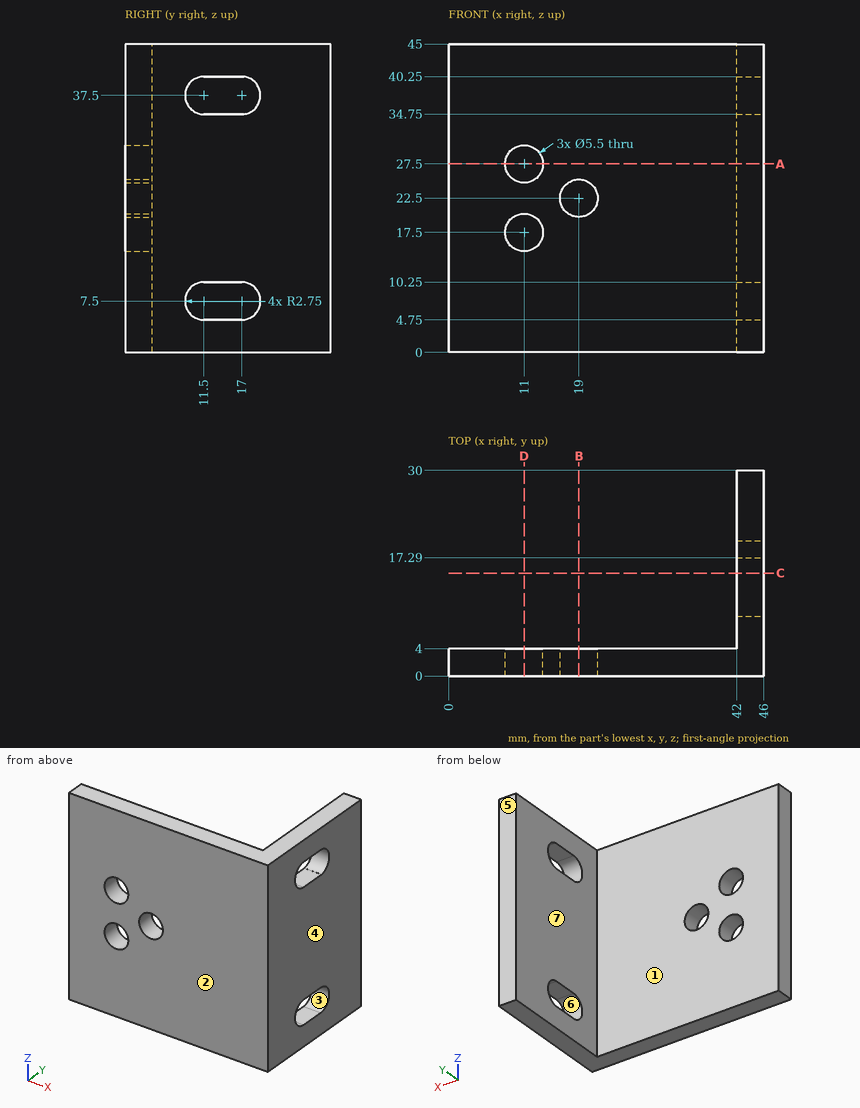
Part print with two shaded views. Sizes in mm from the minimum x, y, z corner. A direction names the side the tool comes from. Coordinates: 2 decimals unless noted, no trailing zeros. Write each loop counter-clockwise with the first axis right and the second up, starting at its lowest first coordinate (ties: lowest second). Pieces come first, ordered by that corner, then holes. Notation, with made-up numbers: M 12,20 L 48,20 A15 cw 48,42 Z; hole C -22.75,-14.5 d9. An arc over 180 degrees is marked long. Return JSON: item names as keys, results as strings.
Item 1: Slice it at B-B, the plane x = 19. Write the cut outline in (y, z), and give its area (3 significant figures).
Findings below:
{"outline": "M 0,0 L 4,0 L 4,19.75 L 0,19.75 Z; M 0,25.25 L 4,25.25 L 4,45 L 0,45 Z", "area": "158 mm2"}
Item 2: Two-plate mould, pull along Y, no slides. Class the marked faces 1, 2, 3 and 4: +Y half, -Y half, draft (parallel to the pull), parting line (faces both ways), or undercut.
Findings below:
{"face 1": "+Y half", "face 2": "-Y half", "face 3": "undercut", "face 4": "draft"}
Item 3: Slice it at C-C, the plane y = 15. Write the cut outline in (x, z).
Findings below:
{"outline": "M 42,0 L 46,0 L 46,4.75 L 42,4.75 Z; M 42,10.25 L 46,10.25 L 46,34.75 L 42,34.75 Z; M 42,40.25 L 46,40.25 L 46,45 L 42,45 Z"}
Item 4: Drop flat-ended pins along their axis: pin 1 Ø1.5 at (y, z) = (20, 27) entering from -X; pin 2 Ø3 at (x, z) = (14, 15.5) entering from +Y. Give the stop position or say it passes through.
Findings below:
{"pin 1": "stops at x = 42", "pin 2": "stops at y = 4"}
Item 5: Which spindle directions (+Z, -Z, +X, -X, +Y, -Y) get a long thin tool onto all of the face, cutting with end or side? Do the marked faces 5, 6 and 7. Say none if no direction does.
Findings below:
{"face 5": "+Z, -Z, +X, -X, +Y", "face 6": "+X, -X", "face 7": "+Z, -Z, -X, +Y"}
Item 6: Slice it at D-D, the plane x = 11. Write the cut outline in (y, z), and give its area (3 significant figures).
Findings below:
{"outline": "M 0,0 L 4,0 L 4,14.75 L 0,14.75 Z; M 0,20.25 L 4,20.25 L 4,24.75 L 0,24.75 Z; M 0,30.25 L 4,30.25 L 4,45 L 0,45 Z", "area": "136 mm2"}
Item 7: Slice it at A-A, the plane z = 27.5. Write the cut outline in (x, y).
Findings below:
{"outline": "M 0,0 L 8.25,0 L 8.25,4 L 0,4 Z; M 13.75,0 L 46,0 L 46,30 L 42,30 L 42,4 L 13.75,4 Z"}
Item 8: Probe line 1 (Z direction, x = 11, y = 0.85); line 2 (X direction, y = 1.45, z = 22.5); line 3 (X direction, y = 12, z = 16.5). List the from-to ranges inside material, lowest first. Write a range as from..to.
Findings below:
{"line 1": "z = 0..14.75, 20.25..24.75, 30.25..45", "line 2": "x = 0..16.25, 21.75..46", "line 3": "x = 42..46"}
